Here's how the part is built. I have some questions about the finished solid (model axes, mm). A direction names the side the tool comes from. Round coordinates to 2 decimals unless told otherwise and drop trailing zeros. Loops run counter-clockwise (first coordinate to the right, second up) from the corner with the lowest first, then second, coordinate; pieces in that order, holes last. Notation, with made-up numbers: M 18,65 L 72,65 A18 cw 72,100 Z; hole C 30.5,54 d1. An arc over 180 degrees is marked long. Answer as a JSON object with one key per item and string values.
from build123d import *

# Parameters (mm, degrees)
EXTRUDE_1_DEPTH     = 15
SKETCH_2_R          = 1.5
CUT_EXTRUDE_1_DEPTH = 15
SKETCH_3_R          = 1.5
CUT_EXTRUDE_2_DEPTH = 45.395945761
FILLET_1_R          = 2.5


with BuildPart() as part:
    # 草图1 → 凸台-拉伸1 (new body)
    with BuildSketch(Plane.XY):
        Polygon((19.5, 0), (-19.5, 0), (-19.5, 15), (-16.5, 15), (-16.5, 3), (-12.5, 3), (-12.5, 15), (-10.5, 15), (-10.5, 3), (10.5, 3), (10.5, 15), (12.5, 15), (12.5, 3), (16.5, 3), (16.5, 15), (19.5, 15), align=None)
    extrude(amount=EXTRUDE_1_DEPTH)

    # 草图2 → 切除-拉伸1 (cut)
    with BuildSketch(Plane(origin=(0, 3, 0), x_dir=(1, 0, 0), z_dir=(0, 1, 0))):
        with Locations(Location((-4, -7.5, 0), (0, 0, 270))):
            Circle(SKETCH_2_R)
        with Locations(Location((4, -7.5, 0), (0, 0, 270))):
            Circle(SKETCH_2_R)
    extrude(amount=-CUT_EXTRUDE_1_DEPTH, mode=Mode.SUBTRACT)

    # 草图3 → 切除-拉伸2 (cut, through all)
    with BuildSketch(Plane(origin=(19.5, 0, 0), x_dir=(0, 0, -1), z_dir=(1, 0, 0))):
        with Locations(Location((-12, 9, 0), (0, 0, 90))):
            Circle(SKETCH_3_R)
        with Locations(Location((-3, 9, 0), (0, 0, 270))):
            Circle(SKETCH_3_R)
    extrude(amount=-CUT_EXTRUDE_2_DEPTH, mode=Mode.SUBTRACT)

    # 圆角1
    fillet_1_edges = [part.edges().sort_by_distance(p)[0] for p in [
        (-10.5, 3, 7.5),
        (10.5, 3, 7.5),
    ]]
    fillet(fillet_1_edges, radius=FILLET_1_R)


solid = part.part
Item 1: For P1, Ø3.5, axis at x = -4, z = 7.5, coming from the +Y side; P2, Ø3, axis at x = -9.5, z = 8.5, coming from the +Y side; P3, Ø2.5, axis at x = 4, z = 7.5, coming from the +Y side, each with a flat end and sliding along its axis, tell me the tip position at first contact or that it passes through.
Solution:
{"P1": "stops at y = 3", "P2": "stops at y = 15", "P3": "passes through"}
Item 2: For faces 1 (the face through (0.3, 2.6, 15)), 2 (the face through (-10.5, 10, 7)), which set-ups out of +Z, -Z, +X, -X, +Y, -Y let a thin tool reach every point of the face, with its end or its side?
Solution:
{"face 1": "+Z, +X, -X, +Y, -Y", "face 2": "+Z, -Z, +Y"}
Item 3: We'd pull the mould along Y, two halves only. Please class faces 3 (the face through (11.51, 7.5, 12.07)), 4 (the face through (18, 15, 7)), 5 (the face through (-16.5, 9, 7)): +Y half, -Y half, draft (parallel to the pull), parting line (faces both ways), or undercut.
Solution:
{"face 3": "undercut", "face 4": "+Y half", "face 5": "draft"}
Item 4: I want a section at A-A on x = 4. List the corners of the cut face in (y, z) for me.
Solution:
{"outline": "M 0,0 L 3,0 L 3,6 L 0,6 Z; M 0,9 L 3,9 L 3,15 L 0,15 Z"}
Item 5: I want a section at B-B on z = 3. Count the separate pieces of the cut face and the enclosed holes in it, plus the area to 3 significant figures.
Solution:
{"separate pieces": "5", "enclosed holes": "0", "area": "210 mm2"}
Item 6: If I drill on L1, parallel to X at y = 12.5, z = 1; L2, parallel to Z at x = 12.05, y = 9; L3, parallel to Y at x = -6, z = 12.75, over which ranges is the centre line in solid material (lowest first)? Write a range as from..to.
Solution:
{"L1": "x = -19.5..-16.5, -12.5..-10.5, 10.5..12.5, 16.5..19.5", "L2": "z = 0..1.5, 4.5..10.5, 13.5..15", "L3": "y = 0..3"}
Item 7: I want a section at C-C on z = 7.5. List the corners of the cut face in (x, y) for me.
Solution:
{"outline": "M -19.5,0 L -5.5,0 L -5.5,3 L -8,3 A2.5 cw -10.5,5.5 L -10.5,15 L -12.5,15 L -12.5,3 L -16.5,3 L -16.5,15 L -19.5,15 Z; M -2.5,0 L 2.5,0 L 2.5,3 L -2.5,3 Z; M 5.5,0 L 19.5,0 L 19.5,15 L 16.5,15 L 16.5,3 L 12.5,3 L 12.5,15 L 10.5,15 L 10.5,5.5 A2.5 cw 8,3 L 5.5,3 Z"}
